from build123d import *

# Parameters (mm, degrees)
ESBO_O1_W                   = 14.3
ESBO_O1_H                   = 31
ESBO_O1_R                   = 1.55
RESSALTO_EXTRUS_O1_DEPTH    = 1.55
ESBO_O2_W                   = 6.85
ESBO_O2_H                   = 6.85
RESSALTO_EXTRUS_O2_DEPTH    = 6.45
ESBO_O3_R                   = 1.65
CORTE_EXTRUS_O1_DEPTH       = 0.5
ESBO_O4_W                   = 7.3
ESBO_O4_H                   = 2.5
RESSALTO_EXTRUS_O3_DEPTH    = 4.05
RESSALTO_EXTRUS_O4_DEPTH    = 1
RESSALTO_EXTRUS_O4_2_DEPTH  = 1
ESBO_O6_R                   = 2.5
RESSALTO_EXTRUS_O5_DEPTH    = 8.8
FILETE1_R                   = 2.5
FILETE2_R                   = 2.5
RESSALTO_EXTRUS_O6_DEPTH    = 13.8
ESBO_O9_R                   = 1.55
CORTE_EXTRUS_O3_DEPTH       = 0.2
CORTE_EXTRUS_O2_START       = -2.2
CORTE_EXTRUS_O2_OUTLINE_W   = 1.65
CORTE_EXTRUS_O2_OUTLINE_H   = 3.08301819
CORTE_EXTRUS_O2_OUTLINE_W_2 = 2
CORTE_EXTRUS_O2_OUTLINE_W_3 = 4
CORTE_EXTRUS_O2_OUTLINE_W_4 = 2.15
CORTE_EXTRUS_O2_DEPTH       = 2.2
RESSALTO_EXTRUS_O7_START    = -7.3
RESSALTO_EXTRUS_O7_DEPTH    = 7.3
ESBO_O12_W                  = 1.34798559
ESBO_O12_H                  = 5.991047065
ESBO_O12_W_2                = 0.998507844
ESBO_O12_W_3                = 2
CORTE_EXTRUS_O4_DEPTH       = 2.2


# Read off the part's stored shape, not the designer's step: Corte-extrus_o2, Ressalto-extrus_o7
with BuildPart() as part:
    # Esbo_o1 → Ressalto-extrus_o1 (new body)
    with BuildSketch(Plane.XY):
        Rectangle(ESBO_O1_W, ESBO_O1_H)
        with Locations(Location((0, -8.5, 0), (0, 0, 180))):
            Circle(ESBO_O1_R, mode=Mode.SUBTRACT)
    extrude(amount=RESSALTO_EXTRUS_O1_DEPTH)

    # Esbo_o2 → Ressalto-extrus_o2 (add)
    with BuildSketch(Plane.XY):
        with Locations((3.525, 0.5664641)):
            Rectangle(ESBO_O2_W, ESBO_O2_H)
    extrude(amount=RESSALTO_EXTRUS_O2_DEPTH)

    # Esbo_o3 → Corte-extrus_o1 (cut)
    with BuildSketch(Plane.XY.offset(6.45)):
        with Locations((3.525, 0.5664641)):
            Circle(ESBO_O3_R)
        with BuildLine():
            Line((3.775, 0.8164641), (3.775, 2.096169954))
            ThreePointArc((3.775, 2.096169954), (4.621015511, 1.662479611), (5.054705854, 0.8164641))
            Line((5.054705854, 0.8164641), (3.775, 0.8164641))
        make_face(mode=Mode.SUBTRACT)
        with BuildLine():
            Line((3.775, -0.963241754), (3.775, 0.3164641))
            Line((3.775, 0.3164641), (5.054705854, 0.3164641))
            ThreePointArc((5.054705854, 0.3164641), (4.621015511, -0.529551411), (3.775, -0.963241754))
        make_face(mode=Mode.SUBTRACT)
        with BuildLine():
            Line((3.275, -0.963241754), (3.275, 0.3164641))
            Line((3.275, 0.3164641), (1.995294146, 0.3164641))
            ThreePointArc((1.995294146, 0.3164641), (2.428984489, -0.529551411), (3.275, -0.963241754))
        make_face(mode=Mode.SUBTRACT)
        with BuildLine():
            Line((3.275, 0.8164641), (3.275, 2.096169954))
            ThreePointArc((3.275, 2.096169954), (2.428984489, 1.662479611), (1.995294146, 0.8164641))
            Line((1.995294146, 0.8164641), (3.275, 0.8164641))
        make_face(mode=Mode.SUBTRACT)
    extrude(amount=-CORTE_EXTRUS_O1_DEPTH, mode=Mode.SUBTRACT)

    # Esbo_o4 → Ressalto-extrus_o3 (add)
    with BuildSketch(Plane.XY):
        with Locations((0, -14.15)):
            Rectangle(ESBO_O4_W, ESBO_O4_H)
    extrude(amount=RESSALTO_EXTRUS_O3_DEPTH)



with BuildPart() as body_2:
    # Esbo_o5 → Ressalto-extrus_o4 (new body)
    with BuildSketch(Plane(origin=(0, 16.5, 0), x_dir=(1, 0, 0), z_dir=(0, 1, 0))):
        with BuildLine():
            Line((1, -5.019693846), (1, -2.080306154))
            ThreePointArc((1, -2.080306154), (6.4, -3.55), (1, -5.019693846))
        make_face()
    extrude(amount=RESSALTO_EXTRUS_O4_DEPTH)



with BuildPart() as body_3:
    # Esbo_o5 → Ressalto-extrus_o4 2 (new body)
    with BuildSketch(Plane(origin=(0, 16.5, 0), x_dir=(1, 0, 0), z_dir=(0, 1, 0))):
        with BuildLine():
            Line((-6, -2.080306154), (-6, -5.019693846))
            ThreePointArc((-6, -5.019693846), (-0.6, -3.55), (-6, -2.080306154))
        make_face()
    extrude(amount=RESSALTO_EXTRUS_O4_2_DEPTH)


with BuildPart() as body_2_1:
    add(body_2.part)

    add(body_3.part)  # Ressalto-extrus_o5 merges body 3
    # Esbo_o6 → Ressalto-extrus_o5 (add)
    with BuildSketch(Plane(origin=(0, 16.5, 0), x_dir=(1, 0, 0), z_dir=(0, 1, 0))):
        with Locations(Location((3.5, -3.55, 0), (0, 0, 180))):
            Circle(ESBO_O6_R)
        with Locations(Location((-3.5, -3.55, 0), (0, 0, 180))):
            Circle(ESBO_O6_R)
    extrude(amount=RESSALTO_EXTRUS_O5_DEPTH)

    # Filete1
    filete1_edges = [body_2_1.edges().sort_by_distance(p)[0] for p in [
        (-1, 25.3, 3.55),
    ]]
    fillet(filete1_edges, radius=FILETE1_R)

    # Filete2
    filete2_edges = [body_2_1.edges().sort_by_distance(p)[0] for p in [
        (6, 25.3, 3.55),
    ]]
    fillet(filete2_edges, radius=FILETE2_R)


with BuildPart() as part_1:
    add(part.part)

    add(body_2_1.part)  # Ressalto-extrus_o6 merges body 2
    # Esbo_o7 → Ressalto-extrus_o6 (add)
    with BuildSketch(Plane.ZY.offset(7.15)):
        with BuildLine():
            Line((3.35, 16.5), (3.35, 14.11698181))
            ThreePointArc((3.35, 14.11698181), (3.262132034, 13.904849775), (3.05, 13.81698181))
            Line((3.05, 13.81698181), (1.55, 13.81698181))
            Line((1.55, 13.81698181), (1.55, 13.41698181))
            Line((1.55, 13.41698181), (3.05, 13.41698181))
            ThreePointArc((3.05, 13.41698181), (3.544974747, 13.622007063), (3.75, 14.11698181))
            Line((3.75, 14.11698181), (3.75, 16.5))
            Line((3.75, 16.5), (3.35, 16.5))
        make_face()
    extrude(amount=-RESSALTO_EXTRUS_O6_DEPTH)

    # Esbo_o9 → Corte-extrus_o3 (cut)
    with BuildSketch(Plane.XY.offset(6.45)):
        with Locations((3.525, 0.5664641)):
            Circle(ESBO_O9_R)
    extrude(amount=-CORTE_EXTRUS_O3_DEPTH, mode=Mode.SUBTRACT)

    # Corte-extrus_o2 outline → Corte-extrus_o2 (cut)
    with BuildSketch(Plane.XY.offset(3.75).offset(CORTE_EXTRUS_O2_START)):
        with Locations((5.825, 14.958490905)):
            Rectangle(CORTE_EXTRUS_O2_OUTLINE_W, CORTE_EXTRUS_O2_OUTLINE_H)
        with Locations((3.5, 14.958490905)):
            Rectangle(CORTE_EXTRUS_O2_OUTLINE_W_2, CORTE_EXTRUS_O2_OUTLINE_H)
        with Locations((0, 14.958490905)):
            Rectangle(CORTE_EXTRUS_O2_OUTLINE_W_3, CORTE_EXTRUS_O2_OUTLINE_H)
        with Locations((-3.5, 14.958490905)):
            Rectangle(CORTE_EXTRUS_O2_OUTLINE_W_2, CORTE_EXTRUS_O2_OUTLINE_H)
        with Locations((-6.075, 14.958490905)):
            Rectangle(CORTE_EXTRUS_O2_OUTLINE_W_4, CORTE_EXTRUS_O2_OUTLINE_H)
    extrude(amount=CORTE_EXTRUS_O2_DEPTH, mode=Mode.SUBTRACT)

    # Ressalto-extrus_o7 outline → Ressalto-extrus_o7 (add)
    with BuildSketch(Plane.ZY.offset(3.65).offset(RESSALTO_EXTRUS_O7_START)):
        with BuildLine():
            ThreePointArc((5.167357012, -14.65), (4.962331759, -14.155025253), (4.467357012, -13.95))
            Line((4.467357012, -13.95), (4.05, -13.95))
            Line((4.05, -13.95), (4.05, -14.35))
            Line((4.05, -14.35), (4.467357012, -14.35))
            ThreePointArc((4.467357012, -14.35), (4.679489046, -14.437867966), (4.767357012, -14.65))
            Line((4.767357012, -14.65), (4.767357012, -18.595051461))
            Line((4.767357012, -18.595051461), (5.167357012, -18.595051461))
            Line((5.167357012, -18.595051461), (5.167357012, -14.65))
        make_face()
    extrude(amount=RESSALTO_EXTRUS_O7_DEPTH)

    # Esbo_o12 → Corte-extrus_o4 (cut)
    with BuildSketch(Plane.XY.offset(4.05)):
        with Locations((-3.423992795, -16.372351479)):
            Rectangle(ESBO_O12_W, ESBO_O12_H)
        with Locations((3.249253922, -16.372351479)):
            Rectangle(ESBO_O12_W_2, ESBO_O12_H)
        with Locations((-1.25, -16.372351479)):
            Rectangle(ESBO_O12_W_3, ESBO_O12_H)
        with Locations((1.25, -16.372351479)):
            Rectangle(ESBO_O12_W_3, ESBO_O12_H)
    extrude(amount=CORTE_EXTRUS_O4_DEPTH, mode=Mode.SUBTRACT)


solid = part_1.part
For this review, take the finished solid that the model builds, in its own axes (mm). A direction names the side the tool comes from. Give positions to 0.01 mm unless a question says otherwise; leave off trailing zeros. Loops run counter-clockwise (first coordinate to the right, second up) from the corner with the lowest first, then second, coordinate; pieces in that order, holes last.
Item 1: Take a section at A-A, the plane y = -8.5. State the section outline as (x, z) points, and give its area (3 significant figures).
Item 2: Insertion check: pin 1 (1.2 mm diameter, centred on y = -16, z = 5, fed in from +X); pin 2 (5 mm diameter, centred on x = 1, y = -12, fed in from +Z); pin 3 (1 mm diameter, centred on y = 17.5, z = 1.5, fed in from +X). Each pin has a flat end and moves straight along its axis. Give the tip position at first contact, or say it passes through.
Item 3: Draft analysis for pull direction Y (two halves, no side actions). For faces 4 (the flat face through (0, -15.5, 1)), 5 (the flat face through (4, 16.5, 4)), 6 (the flat face through (0.1, 1, 4)), state which applies: +Y half, -Y half, draft (parallel to the pull), parting line (faces both ways), or undercut.
Item 4: Take a section at B-B, the plane y = 19.5. State the section outline as (x, z) points, and give its area (3 significant figures).
Item 5: For line 1 along X through (y, z) = (-8.5, 0.7); line 2 along Y through (x, z) = (-2.25, 1); line 3 along Y through (x, z) = (3.5, 3.5), list the stretches that pass through material, from the lowest coordinate up.
Item 6: Tool access review of faces 1 (the flat face through (3, 1, 6.25)), 2 (the flat face through (0, -12.9, 3)), 3 (the flat face through (-0.25, -16, 5)): name each direction out of +Z, -Z, +X, -X, +Y, -Y from which nothing blocks a thin tool from reaching the whole face with its end or side.
Calculated:
1. outline: (-7.15, 0) - (-1.55, 0) - (-1.55, 1.55) - (-7.15, 1.55) - close; (1.55, 0) - (7.15, 0) - (7.15, 1.55) - (1.55, 1.55) - close
1. area: 17.4 mm2
2. pin 1: stops at x = 2.75
2. pin 2: stops at z = 5.12
2. pin 3: stops at x = 5.95
3. face 4: -Y half
3. face 5: undercut
3. face 6: draft
4. outline: circle Ø5 at (-3.5, 3.55); circle Ø5 at (3.5, 3.55)
4. area: 39.3 mm2
5. line 1: x = -7.15 to -1.55, 1.55 to 7.15
5. line 2: y = -15.5 to 15.5, 16.5 to 17.5
5. line 3: y = -15.4 to -12.9, -2.86 to 3.99, 16.5 to 25.3
6. face 1: +Z
6. face 2: +Z, +X, -X
6. face 3: +Z, +Y, -Y
